Autodesk Inventor part; units mm, degrees
ref_plane "YZ Plane" through (0, 0, 0) normal (1, 0, 0) x (0, 1, 0)
ref_plane "XZ Plane" through (0, 0, 0) normal (0, 1, 0) x (-1, 0, 0)
ref_plane "XY Plane" through (0, 0, 0) normal (0, 0, 1) x (1, 0, 0)
sketch "Эскиз1" plane through (0, 0, 0) normal (0, 0, 1) x (1, 0, 0)
  line L0 (10, 0) -> (30, 0)
  line L1 (30, 0) -> (40, 24)
  line L2 (10, 0) -> (0, 24)
  circle A0 centre (20, 8) radius 4
  line L3 (0, 24) -> (40, 24)
  point P0 (0, 0)
  dimension "d0" = 24
  dimension "d1" = 40
  dimension "d3" = 20
  dimension "d6" = 8
extrude "Выдавливание1" add sketch "Эскиз1" along normal blind 10
properties part number "N2"
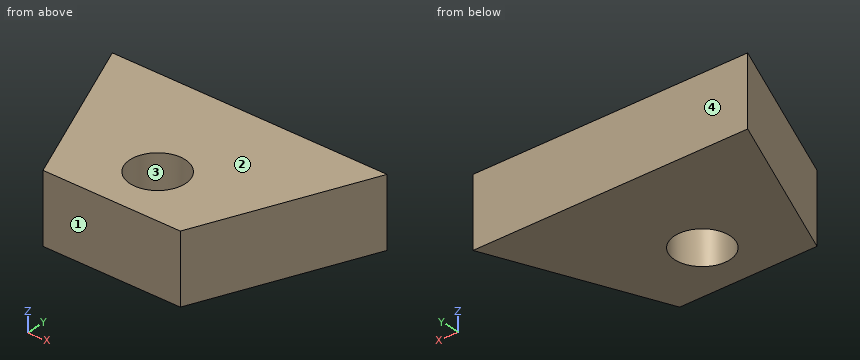
Geometry: final body of the model. Coordinates: model frame, mm. Face numbers are marked on the shaded views. Round coordinates to 2 decimals unless told otherwise and drop trailing zeros. Order: outer loops, then holes, each group sorted by start corner. A loop starts at its lowest first (then second) coordinate and runs counter-clockwise, first axis right, second up. Notation, with made-up numbers: (45.5, 78.25) -> (51.5, 78.25) arc R15 cw to (51.5, 93.25) -> close; hole circle Ø9 at (72, 81). An arc over 180 degrees is marked (long way). Use CSV: the item, a comma, the result in double quotes. Start each with the question number.
1) First-contact query: pin 1 Ø3 at (y, z) = (14.5, 3.5) entering from -X; pin 2 Ø6 at (y, z) = (15, 6) entering from -X. Flat tips, straight axial feed; report the tip coordinate or a pass-through.
2) Section D-D (x = 37). Return the cut outline in (y, z), and give its area (3 significant figures).
3) Draft query along Y for the marked faces 1, 2, 3 and 4. Return one class per face: +Y half, -Y half, draft (parallel to the pull), parting line (faces both ways), or undercut.
4) Material intervals for line 1 along Y through (x, z) = (20, 5.25); line 2 along X through (y, z) = (11, 1); line 3 along Y through (x, z) = (18.5, 9.25), sorted ascending. Write a range as from..to.
5) Section C-C (y = 8). Return the cut outline in (x, z), and give its area (3 significant figures).
6) Section B-B (x = 20). Return the cut outline in (y, z), and give its area (3 significant figures).
7) Section A-A (z = 7.75). Return the cut outline in (x, y), and give its area (3 significant figures).
Returned:
1,pin 1,"stops at x = 3.33"
1,pin 2,"stops at x = 2.5"
2,outline,"(16.8, 0) -> (24, 0) -> (24, 10) -> (16.8, 10) -> close"
2,area,"72.0 mm²"
3,face 1,"-Y half"
3,face 2,"draft"
3,face 3,"undercut"
3,face 4,"+Y half"
4,line 1,"y = 0..4, 12..24"
4,line 2,"x = 5.42..17.35, 22.65..34.58"
4,line 3,"y = 0..4.29, 11.71..24"
5,outline,"(6.67, 0) -> (16, 0) -> (16, 10) -> (6.67, 10) -> close; (24, 0) -> (33.33, 0) -> (33.33, 10) -> (24, 10) -> close"
5,area,"187 mm²"
6,outline,"(0, 0) -> (4, 0) -> (4, 10) -> (0, 10) -> close; (12, 0) -> (24, 0) -> (24, 10) -> (12, 10) -> close"
6,area,"160 mm²"
7,outline,"(0, 24) -> (10, 0) -> (30, 0) -> (40, 24) -> close; hole circle Ø8 at (20, 8)"
7,area,"670 mm²"
